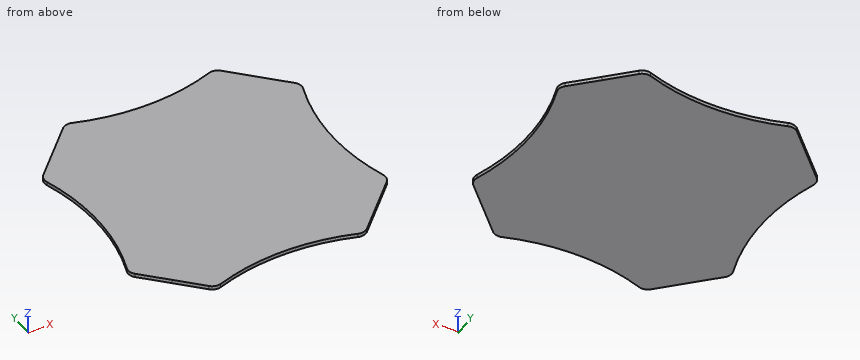
```python
from build123d import *

# Parameters (mm, degrees)
F2_DEPTH = 1.5
F3_R     = 4


with BuildPart() as f2:
    # F1 (on Top) → F2 (new body)
    with BuildSketch(Plane.XY):
        with BuildLine():
            Line((-30.228815, 52.856232), (-41.542523, 41.542523))
            Line((-41.542523, 41.542523), (-52.856232, 30.228815))
            ThreePointArc((-52.856232, 30.228815), (-47.356232, 0), (-52.856232, -30.228815))
            Line((-52.856232, -30.228815), (-41.542523, -41.542523))
            Line((-41.542523, -41.542523), (-30.228815, -52.856232))
            ThreePointArc((-30.228815, -52.856232), (0, -47.356232), (30.228815, -52.856232))
            Line((30.228815, -52.856232), (41.542523, -41.542523))
            Line((41.542523, -41.542523), (52.856232, -30.228815))
            ThreePointArc((52.856232, -30.228815), (47.356232, 0), (52.856232, 30.228815))
            Line((52.856232, 30.228815), (41.542523, 41.542523))
            Line((41.542523, 41.542523), (30.228815, 52.856232))
            ThreePointArc((30.228815, 52.856232), (0, 47.356232), (-30.228815, 52.856232))
        make_face()
    extrude(amount=F2_DEPTH)

    # F3
    f3_edges = [f2.edges().sort_by_distance(p)[0] for p in [
        (-52.856232, 30.228815, 0.75),
        (-30.228815, 52.856232, 0.75),
        (30.228815, 52.856232, 0.75),
        (52.856232, 30.228815, 0.75),
        (52.856232, -30.228815, 0.75),
        (30.228815, -52.856232, 0.75),
        (-30.228815, -52.856232, 0.75),
        (-52.856232, -30.228815, 0.75),
    ]]
    fillet(f3_edges, radius=F3_R)


solid = f2.part
```
The listing builds one solid part. Answer for the finished solid, in the listing's coordinates (mm). Give positions to 0.01 mm unless a question says otherwise; leave off trailing zeros. Loops run counter-clockwise (first coordinate to the right, second up) from the corner with the lowest first, then second, coordinate; pieces in that order, holes last. Notation, with made-up numbers: M -28,32.25 L 28,32.25 A15 cw 28,49.25 Z; hole C -36.5,13.5 d2. An arc over 180 degrees is marked long. One line per item, written item: value.
1. Section C-C on x = -20 is taken. Determine the outline of the cut face in (y, z), plus the area to 3 significant figures.
Found:
outline: M -49.72,0 L 49.72,0 L 49.72,1.5 L -49.72,1.5 Z
area: 149 mm^2
2. Section B-B on y = 12 is taken. Determine the outline of the cut face in (x, z).
Found:
outline: M -48.2,0 L 48.2,0 L 48.2,1.5 L -48.2,1.5 Z
3. Section A-A on z = 0.5 is taken. Determine the outline of the cut face in (x, y).
Found:
outline: M -52.02,-27.89 A4 ccw -51.06,-32.02 L -32.02,-51.06 A4 ccw -27.89,-52.02 A85.82 cw 27.89,-52.02 A4 ccw 32.02,-51.06 L 51.06,-32.02 A4 ccw 52.02,-27.89 A85.82 cw 52.02,27.89 A4 ccw 51.06,32.02 L 32.02,51.06 A4 ccw 27.89,52.02 A85.82 cw -27.89,52.02 A4 ccw -32.02,51.06 L -51.06,32.02 A4 ccw -52.02,27.89 A85.82 cw Z
4. Find the intervals of material crossed by probe 1 along X at (y, z) = (-1, 0.65); probe 2 along X at (y, z) = (-40.5, 0.7); probe 3 along Y at (x, z) = (-32.5, 0.2), in increasing order.
Found:
probe 1: -47.36 to 47.36
probe 2: -42.59 to 42.59
probe 3: -50.59 to 50.59
